Read the model definition and answer for the solid it produces. Units are mm, in the model's axes. A direction names the side the tool comes from. Give positions to 0.01 mm unless a question says otherwise; leave off trailing zeros. Write each loop counter-clockwise with the first axis right and the second up, starting at its lowest first coordinate (ties: lowest second). Pieces come first, ordered by that corner, then holes. Notation, with made-up numbers: M 67.5,-17.5 L 81.5,-17.5 A26 ccw 81.5,5.5 Z; hole C 38,18 d3. An arc over 180 degrees is marked long. Use a Markdown table: item, result. Add a question column.
Item 1: Consider probe 1 along X at (y, z) = (-96.5, 569); probe 2 along Z at (x, y) = (-552.5, -9.5); probe 3 along Z at (x, y) = (210, -202.5). Determine where each line is inside the solid, lowest interval first. Write a range as [from, to].
Item 2: A cutting plane is placed at B-B on z = 492. Count the separate pieces of the cut face and the enclosed holes in it, then the cut area to 3 significant figures.
Item 3: The mould has two halves that part along Z. Classify faces 1 (the flat face through (453, -92, 795)), 2 (the flat face through (453, -92, -745)), 3 (the flat face through (-413, -102, 865)), 4 (the flat face through (605, -207, 4)): pulls with the +Z half, pulls with the -Z half, needs draft (parallel to the pull), parting line crosses it, or undercut.
Item 4: For faces 5 (the flat face through (501, -202, -725)), 6 (the flat face through (-406, 20, -4)), 7 (the flat face through (-504, 1, 775)), determine the directions among +Z, -Z, +X, -X, +Y, -Y from which every point of the face is accessible in a straight line to the end or side of a thin tool.
Item 5: Given P1, Ø6, axis at y = -214.5, z = -93.5, coming from the -X side; P2, Ø16, axis at x = -86.5, y = -210.5, coming from the -Z side; P3, Ø1, axis at y = -100, z = -492, coming from the +X side, each flat-ended and moving along its own axis, determine where each tip first touches the part or whether it passes through.
Item 6: A cutting plane is placed at A-A on x = 239. Determine the outline of the cut face in (y, z).
from build123d import *

# Parameters (mm, degrees)
SKETCH1_W           = 20
SKETCH1_H           = 1730
SKETCH1_W_2         = 165
SKETCH1_H_2         = 20
SKETCH1_W_3         = 800
BOSS_EXTRUDE1_DEPTH = 20
LPATTERN1_COUNT     = 2
LPATTERN1_PITCH     = 220
SKETCH2_W           = 20.11323458
SKETCH2_H           = 20
SKETCH2_W_2         = 20
SKETCH2_H_2         = 20.786356151
SKETCH2_W_3         = 20.945730737
SKETCH2_W_4         = 20.439611237
BOSS_EXTRUDE2_DEPTH = 200
SKETCH3_W           = 20
SKETCH3_H           = 100
SKETCH3_H_2         = 50
BOSS_EXTRUDE3_DEPTH = 20
SKETCH4_W           = 20
SKETCH4_H           = 200
BOSS_EXTRUDE4_DEPTH = 20
LPATTERN2_COUNT     = 2
LPATTERN2_PITCH     = 1520
SKETCH5_W           = 20
SKETCH5_H           = 20
BOSS_EXTRUDE5_DEPTH = 1500


with BuildPart() as part:
    # Sketch1 → Boss-Extrude1 (new body)
    with BuildSketch(Plane(origin=(0, 0, 0), x_dir=(1, 0, 0), z_dir=(0, 1, 0))):
        with Locations((-595, 0)):
            Rectangle(SKETCH1_W, SKETCH1_H)
        with Locations((-410, 0)):
            Rectangle(SKETCH1_W, SKETCH1_H)
        with Locations((-502.5, 735)):
            Rectangle(SKETCH1_W_2, SKETCH1_H_2)
        with Locations((-502.5, 855)):
            Rectangle(SKETCH1_W_2, SKETCH1_H_2)
        with Locations((0, 735)):
            Rectangle(SKETCH1_W_3, SKETCH1_H_2)
        with Locations((0, 855)):
            Rectangle(SKETCH1_W_3, SKETCH1_H_2)
        with Locations((502.5, 855)):
            Rectangle(SKETCH1_W_2, SKETCH1_H_2)
        with Locations((410, 0)):
            Rectangle(SKETCH1_W, SKETCH1_H)
        with Locations((502.5, 735)):
            Rectangle(SKETCH1_W_2, SKETCH1_H_2)
        with Locations((595, 0)):
            Rectangle(SKETCH1_W, SKETCH1_H)
        with Locations((502.5, -785)):
            Rectangle(SKETCH1_W_2, SKETCH1_H_2)
        with Locations((502.5, -855)):
            Rectangle(SKETCH1_W_2, SKETCH1_H_2)
        with Locations((-502.5, -785)):
            Rectangle(SKETCH1_W_2, SKETCH1_H_2)
        with Locations((-502.5, -855)):
            Rectangle(SKETCH1_W_2, SKETCH1_H_2)
    extrude(amount=BOSS_EXTRUDE1_DEPTH)


with BuildPart() as lpattern1_1:
    # LPattern1: pattern copy
    add(part.part.moved(Location(Vector(0, -1, 0) * (1 * LPATTERN1_PITCH))))


with BuildPart() as part_1:
    add(part.part)

    add(lpattern1_1.part)  # Boss-Extrude2 merges LPattern1_1
    # Sketch2 → Boss-Extrude2 (add)
    with BuildSketch(Plane(origin=(0, 0, 0), x_dir=(1, 0, 0), z_dir=(0, 1, 0))):
        with Locations((-595.05661729, 735)):
            Rectangle(SKETCH2_W, SKETCH2_H)
        with Locations((-595, 855)):
            Rectangle(SKETCH2_W_2, SKETCH2_H)
        with Locations((-410, 855.393178076)):
            Rectangle(SKETCH2_W_2, SKETCH2_H_2)
        with Locations((-595.472865369, -785)):
            Rectangle(SKETCH2_W_3, SKETCH2_H)
        with Locations((-410, 735)):
            Rectangle(SKETCH2_W_2, SKETCH2_H)
        with Locations((-595, -855)):
            Rectangle(SKETCH2_W_2, SKETCH2_H)
        with Locations((-410, -855)):
            Rectangle(SKETCH2_W_2, SKETCH2_H)
        with Locations((-409.780194381, -785)):
            Rectangle(SKETCH2_W_4, SKETCH2_H)
        with Locations((595.472865369, -785)):
            Rectangle(SKETCH2_W_3, SKETCH2_H)
        with Locations((410, -855)):
            Rectangle(SKETCH2_W_2, SKETCH2_H)
        with Locations((595, -855)):
            Rectangle(SKETCH2_W_2, SKETCH2_H)
        with Locations((410, 735)):
            Rectangle(SKETCH2_W_2, SKETCH2_H)
        with Locations((410, 855.393178076)):
            Rectangle(SKETCH2_W_2, SKETCH2_H_2)
        with Locations((595.05661729, 735)):
            Rectangle(SKETCH2_W, SKETCH2_H)
        with Locations((595, 855)):
            Rectangle(SKETCH2_W_2, SKETCH2_H)
        with Locations((409.780194381, -785)):
            Rectangle(SKETCH2_W_4, SKETCH2_H)
    extrude(amount=-BOSS_EXTRUDE2_DEPTH)

    # Sketch3 → Boss-Extrude3 (add)
    with BuildSketch(Plane.XZ.offset(220)):
        with Locations((-472.5, -795)):
            Rectangle(SKETCH3_W, SKETCH3_H)
        with Locations((-532.5, -795)):
            Rectangle(SKETCH3_W, SKETCH3_H)
        with Locations((-472.5, 820)):
            Rectangle(SKETCH3_W, SKETCH3_H_2)
        with Locations((-532.5, 820)):
            Rectangle(SKETCH3_W, SKETCH3_H_2)
        with Locations((532.5, 820)):
            Rectangle(SKETCH3_W, SKETCH3_H_2)
        with Locations((472.5, 820)):
            Rectangle(SKETCH3_W, SKETCH3_H_2)
        with Locations((532.5, -795)):
            Rectangle(SKETCH3_W, SKETCH3_H)
        with Locations((472.5, -795)):
            Rectangle(SKETCH3_W, SKETCH3_H)
    extrude(amount=-BOSS_EXTRUDE3_DEPTH)

    # Sketch4 → Boss-Extrude4 (add)
    with BuildSketch(Plane.XY.offset(-725)):
        with Locations((-447.5, -100)):
            Rectangle(SKETCH4_W, SKETCH4_H)
        with Locations((-557.5, -100)):
            Rectangle(SKETCH4_W, SKETCH4_H)
        with Locations((557.5, -100)):
            Rectangle(SKETCH4_W, SKETCH4_H)
        with Locations((447.5, -100)):
            Rectangle(SKETCH4_W, SKETCH4_H)
    boss_extrude4 = extrude(amount=-BOSS_EXTRUDE4_DEPTH)

    # LPattern2: Boss-Extrude4 ×2
    with Locations(*[(0, 0, i * LPATTERN2_PITCH) for i in range(1, LPATTERN2_COUNT)]):
        add(boss_extrude4)

    # Sketch5 → Boss-Extrude5 (add)
    with BuildSketch(Plane.XY.offset(-725)):
        with Locations((-557.5, -100)):
            Rectangle(SKETCH5_W, SKETCH5_H)
        with Locations((-447.5, -100)):
            Rectangle(SKETCH5_W, SKETCH5_H)
        with Locations((447.5, -100)):
            Rectangle(SKETCH5_W, SKETCH5_H)
        with Locations((557.5, -100)):
            Rectangle(SKETCH5_W, SKETCH5_H)
    extrude(amount=BOSS_EXTRUDE5_DEPTH)


solid = part_1.part
Filled in:
| question | item | result |
|---|---|---|
| 1 | probe 1 | [-567.5, -547.5], [-457.5, -437.5], [437.5, 457.5], [547.5, 567.5] |
| 1 | probe 2 | [-745, -725], [775, 795] |
| 1 | probe 3 | [-865, -845], [-745, -725] |
| 2 | separate pieces | 12 |
| 2 | enclosed holes | 0 |
| 2 | area | 4,800 mm² |
| 3 | face 1 | undercut |
| 3 | face 2 | undercut |
| 3 | face 3 | pulls with the +Z half |
| 3 | face 4 | needs draft |
| 4 | face 5 | -Y |
| 4 | face 6 | +Z, -Z, +X, -X, +Y |
| 4 | face 7 | +Y |
| 5 | P1 | x = -605 |
| 5 | P2 | z = -865 |
| 5 | P3 | x = 567.5 |
| 6 | outline | M -220,-865 L -200,-865 L -200,-845 L -220,-845 Z; M -220,-745 L -200,-745 L -200,-725 L -220,-725 Z; M 0,-865 L 20,-865 L 20,-845 L 0,-845 Z; M 0,-745 L 20,-745 L 20,-725 L 0,-725 Z |
